Geometry check sheet. Reference: the model listing, model coordinates, mm. Face numbers are marked on the shaded views. A direction names the side the tool comes from. Round coordinates to 2 decimals unless told otherwise and drop trailing zeros. Order: outer loops, then holes, each group sorted by start corner. A loop starts at its lowest first (then second) coordinate and runs counter-clockwise, first axis right, second up. Notation, with made-up numbers: (-15, 35.25) -> (17, 35.25) arc R17 ccw to (17, 43.25) -> close; hole circle Ø10 at (-1.75, 73). An arc over 180 degrees is marked (long way). Answer as a JSON object with one key per item and string values. Group by question number.
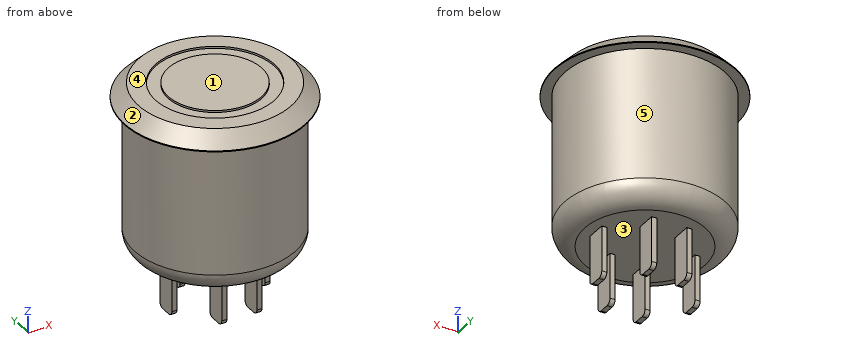
from build123d import *

# Parameters (mm, degrees)
F0_R     = 9
F1_DEPTH = 1.5
F2_SIZE  = 1.4
F3_R     = 5.9
F3_R_2   = 4.65
F4_DEPTH = 0.2
F5_R     = 8
F6_DEPTH = 15
F7_R     = 2
F8_W     = 0.5
F8_H     = 2
F9_DEPTH = 5
F10_R    = 0.5


with BuildPart() as f1:
    # F0 (on Top) → F1 (new body)
    with BuildSketch(Plane.XY):
        Circle(F0_R)
    extrude(amount=F1_DEPTH)

    # F2
    f2_edges = [f1.edges().sort_by_distance(p)[0] for p in [
        (-9, 0, 1.5),
    ]]
    chamfer(f2_edges, length=F2_SIZE)

    # F3 (on face) → F4 (cut)
    with BuildSketch(Plane.XY.offset(1.5)):
        Circle(F3_R)
        Circle(F3_R_2, mode=Mode.SUBTRACT)
    extrude(amount=-F4_DEPTH, mode=Mode.SUBTRACT)

    # F5 (on face) → F6 (join)
    with BuildSketch(Plane(origin=(0, 0, 0), x_dir=(1, 0, 0), z_dir=(0, 0, -1))):
        Circle(F5_R)
    extrude(amount=F6_DEPTH)

    # F7
    f7_edges = [f1.edges().sort_by_distance(p)[0] for p in [
        (-8, 0, -15),
    ]]
    fillet(f7_edges, radius=F7_R)

    # F8 (on face) → F9 (join)
    with BuildSketch(Plane(origin=(0, 0, -15), x_dir=(1, 0, 0), z_dir=(0, 0, -1))):
        with Locations((-1.75, 3.5)):
            Rectangle(F8_W, F8_H)
        with Locations((1.75, 3.5)):
            Rectangle(F8_W, F8_H)
        with Locations((1.75, -3.5)):
            Rectangle(F8_W, F8_H)
        with Locations((-1.75, -3.5)):
            Rectangle(F8_W, F8_H)
        with Locations((-4.65, 0)):
            Rectangle(F8_W, F8_H)
        with Locations((4.65, 0)):
            Rectangle(F8_W, F8_H)
    extrude(amount=F9_DEPTH)

    # F10
    f10_edges = [f1.edges().sort_by_distance(p)[0] for p in [
        (-1.75, -4.5, -20),
        (1.75, -4.5, -20),
        (4.65, -1, -20),
        (-4.65, -1, -20),
        (1.75, 2.5, -20),
        (-1.75, 2.5, -20),
        (-4.65, 1, -20),
        (-1.75, -2.5, -20),
        (1.75, -2.5, -20),
        (4.65, 1, -20),
        (1.75, 4.5, -20),
        (-1.75, 4.5, -20),
    ]]
    fillet(f10_edges, radius=F10_R)


solid = f1.part
Item 1: Sectioned sample at C-C, the plane y = 0. Enter the section's corners in (x, z).
Item 2: Sectioned sample at D-D, the plane z = -7.75. Enter the section's corners in (x, y).
Item 3: Set-up check for the marked faces 4 and 5: record each of +Z, -Z, +X, -X, +Y, -Y from which the full face is reachable in a straight line by a thin tool's end or side.
Item 4: Sectioned sample at A-A, the plane z = -16.5. Enter the section's corners in (x, y).
Item 5: Mould release check, pull along X, two halves, no side actions. Record for the marked faces 1, 2 and 3: pulls with the +X half, pulls with the -X half, needs draft (parallel to the pull), parting line crosses it, or undercut.
Item 6: Sectioned sample at B-B, the plane x = 0. Enter the section's corners in (y, z).
Item 7: Thickness scan on L1, parallel to X at y = 2.75, z = -16.25; L2, parallel to Z at x = -0.5, y = 3.25; L3, parallel to X at y = 4.25, z = -13.5. Record the ranges inside material, lowest first.
Item 8: Depth check by flat-ended pin: pin 1 Ø1 at (y, z) = (0, -18) entering from +X; pin 2 Ø1.5 at (x, z) = (3, -6.5) entering from -Y; pin 3 Ø2 at (x, z) = (0.5, -12.5) entering from -Y. Enter the tip coordinate at first touch or a pass-through.
Result:
{
 "1": {"outline": "(-9, 0) -> (-8, 0) -> (-8, -13) arc R2 ccw to (-6, -15) -> (-4.9, -15) -> (-4.9, -20) -> (-4.4, -20) -> (-4.4, -15) -> (4.4, -15) -> (4.4, -20) -> (4.9, -20) -> (4.9, -15) -> (6, -15) arc R2 ccw to (8, -13) -> (8, 0) -> (9, 0) -> (9, 0.1) -> (7.6, 1.5) -> (5.9, 1.5) -> (5.9, 1.3) -> (4.65, 1.3) -> (4.65, 1.5) -> (-4.65, 1.5) -> (-4.65, 1.3) -> (-5.9, 1.3) -> (-5.9, 1.5) -> (-7.6, 1.5) -> (-9, 0.1) -> close"},
 "2": {"outline": "circle Ø16 at (0, 0)"},
 "3": {"face 4": "+Z, +X, -X, +Y, -Y", "face 5": "-Z"},
 "4": {"outline": "(-4.9, -1) -> (-4.4, -1) -> (-4.4, 1) -> (-4.9, 1) -> close; (-2, -4.5) -> (-1.5, -4.5) -> (-1.5, -2.5) -> (-2, -2.5) -> close; (-2, 2.5) -> (-1.5, 2.5) -> (-1.5, 4.5) -> (-2, 4.5) -> close; (1.5, -4.5) -> (2, -4.5) -> (2, -2.5) -> (1.5, -2.5) -> close; (1.5, 2.5) -> (2, 2.5) -> (2, 4.5) -> (1.5, 4.5) -> close; (4.4, -1) -> (4.9, -1) -> (4.9, 1) -> (4.4, 1) -> close"},
 "5": {"face 1": "needs draft", "face 2": "parting line crosses it", "face 3": "undercut"},
 "6": {"outline": "(-9, 0) -> (-8, 0) -> (-8, -13) arc R2 ccw to (-6, -15) -> (6, -15) arc R2 ccw to (8, -13) -> (8, 0) -> (9, 0) -> (9, 0.1) -> (7.6, 1.5) -> (5.9, 1.5) -> (5.9, 1.3) -> (4.65, 1.3) -> (4.65, 1.5) -> (-4.65, 1.5) -> (-4.65, 1.3) -> (-5.9, 1.3) -> (-5.9, 1.5) -> (-7.6, 1.5) -> (-9, 0.1) -> close"},
 "7": {"L1": "x = -2 to -1.5, 1.5 to 2", "L2": "z = -15 to 1.5", "L3": "x = -6.7 to 6.7"},
 "8": {"pin 1": "stops at x = 4.9", "pin 2": "stops at y = -7.68", "pin 3": "stops at y = -8"}
}
